Geometry: see drawing. Coordinates: mm, zero at the bounding-box minimum. A direction names the side the tool comes from. Round coordinates to 2 decimals unless told otherwise and drop trailing zeros. Loops run counter-clockwise (first coordinate to the right, second up) from the corner with the lowest first, then second, coordinate; pieces in that order, holes last. Notation, with made-up numbers: M 48,-39.75 L 92,-39.75 A18 ccw 92,-16.75 Z; hole C -27.5,-3 d1. An arc over 180 degrees is marked long. Answer as a JSON object with one key per item and string values.
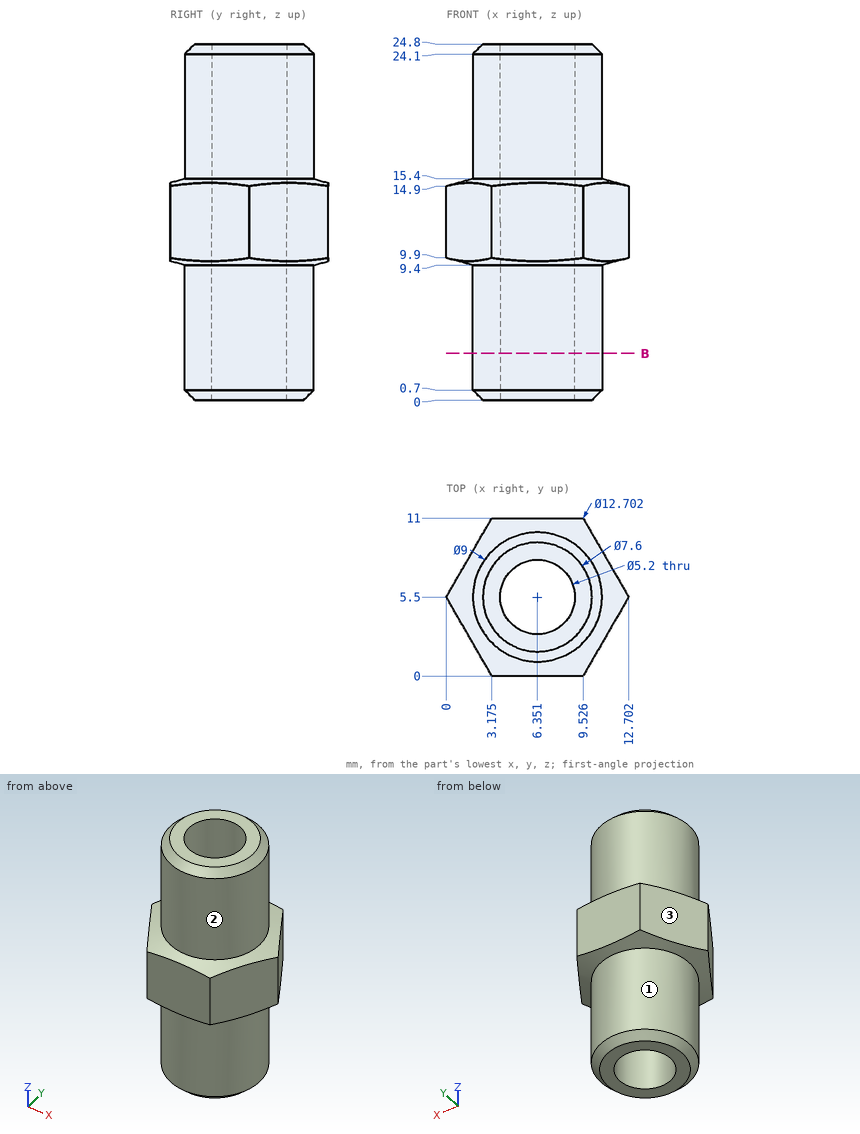
1) Section query B-B (z = 3.25). Return the cut outline in (x, y).
Results:
{"outline": "C 6.35,5.5 d9; hole C 6.35,5.5 d5.2"}
2) Ray query, line 1 (Y direction, x = 5, z = 15); line 2 (Y direction, x = 7.25, z = 7.5); line 3 (X direction, y = 5.75, z = 13.5) (1 decimal). Return the intervals inside material, ascending.
Results:
{"line 1": "0 to 3.28, 7.72 to 11", "line 2": "1.09 to 3.06, 7.94 to 9.91", "line 3": "0.1 to 3.8, 8.9 to 12.6"}
3) Pin query (flat end, axial travel): P1, Ø1, axis at y = 10, z = 8.5, coming from the +X side (1 decimal); P2, Ø4, axis at y = 10, z = 9.5, coming from the +X side (1 decimal); P3, Ø1, axis at y = 8, z = 11, coming from the -X side (1 decimal). Return the tip coordinate at first contact, or that it passes through.
Results:
{"P1": "x = 8.4", "P2": "x = 11.3", "P3": "x = 1.2"}
4) Reachability of the marked faces 1, 2 and 3 from +Z, -Z, +X, -X, +Y, -Y: full face, straight path, thin tool, end or side. Return the list, or none.
Results:
{"face 1": "-Z", "face 2": "+Z", "face 3": "+Z, -Z, -X, +Y"}
